from build123d import *

# Parameters (mm, degrees)
F0_R     = 1.905
F1_DEPTH = 38.1
F2_W     = 71.755
F2_H     = 11.43
F2_R     = 1.905
F3_DEPTH = 0.762
F5_DEPTH = 11.43
F6_R     = 0.762


# Not quite as in the source:
# - a feature names something its author has since deleted; it is built from what else it names


with BuildPart() as f1:
    # F0 (on Top) → F1 (new body)
    with BuildSketch(Plane.XY):
        Circle(F0_R)
    extrude(amount=F1_DEPTH)

    # F2 (on face) → F3 (join)
    with BuildSketch(Plane.XY.offset(38.1)):
        Rectangle(F2_W, F2_H)
        Circle(F2_R, mode=Mode.SUBTRACT)
    extrude(amount=-F3_DEPTH)

    # F4 (on face) → F5 (join, through all)
    with BuildSketch(Plane.XZ.offset(5.715)):
        with BuildLine():
            ThreePointArc((0, 46.1144251321), (-18.0910863279, 47.2907715726), (-35.8775, 50.8))
            Line((-35.8775, 50.8), (-35.8775, 48.0069763479))
            ThreePointArc((-35.8775, 48.0069763479), (-23.5669827894, 41.6891623658), (-10.2035430744, 38.1))
            Line((-10.2035430744, 38.1), (0, 38.1))
            Line((0, 38.1), (0, 46.1144251321))
        make_face()
        with BuildLine():
            ThreePointArc((35.8775, 50.8), (18.0910863279, 47.2907715726), (0, 46.1144251321))
            Line((0, 46.1144251321), (0, 38.1))
            Line((0, 38.1), (10.2035430744, 38.1))
            ThreePointArc((10.2035430744, 38.1), (23.5669827894, 41.6891623658), (35.8775, 48.0069763479))
            Line((35.8775, 48.0069763479), (35.8775, 50.8))
        make_face()
    extrude(amount=-F5_DEPTH)

    # F6
    f6_edges = [f1.edges().sort_by_distance(p)[0] for p in [
        (10.203543, 0, 38.1),
        (-10.203543, 0, 38.1),
    ]]
    fillet(f6_edges, radius=F6_R)


solid = f1.part
Work out the finished part from the listing and answer in its coordinate system (mm). A direction names the side the tool comes from. Give positions to 0.01 mm unless a question says otherwise; leave off trailing zeros. Write each loop counter-clockwise with the first axis right and the second up, starting at its lowest first coordinate (ties: lowest second). Pieces come first, ordered by that corner, then holes.
Q1. A tool of negligible diameter and unlimited length cuts with its end or side. For faces 1 (the face through (26.734, -0.08, 43.007)), 2 (the face through (-0.41, -1.86, 18.41)), 3 (the face through (-35.878, 0, 49)), 4 (the face through (-27, 0, 38.1)), from which of +Z, -Z, +X, -X, +Y, -Y can it reach the whole face along a straight path? Write none if from no direction.
Answer:
face 1: +X, +Y, -Y
face 2: -Z
face 3: +Z, -Z, -X, +Y, -Y
face 4: -X, +Y, -Y
Q2. For a pull along Z with two mould halves and no side action, classify faces 5 (the face through (-1, 5.715, 43)), 6 (the face through (16.637, 0.08, 38.746)), 7 (the face through (0, 0, 0)) as released by +Z, released by -Z, zero draft, split by the parting line, or undercut.
Answer:
face 5: zero draft
face 6: undercut
face 7: released by -Z
Q3. The part is cut by section B-B on x = 19. Give the vertices of the cut face in (y, z) (3 decimals).
Answer:
outline: (-5.715, 37.338) - (5.715, 37.338) - (5.715, 38.1) - (-5.715, 38.1) - close; (-5.715, 40.118) - (5.715, 40.118) - (5.715, 47.413) - (-5.715, 47.413) - close
Q4. The part is cut by section D-D on z = 27. Give the vertices of the cut face in (x, y) (3 decimals).
Answer:
outline: circle Ø3.81 at (0, 0)
Q5. The part is cut by section C-C on x = 28. Give the vertices of the cut face in (y, z) (3 decimals).
Answer:
outline: (-5.715, 37.338) - (5.715, 37.338) - (5.715, 38.1) - (-5.715, 38.1) - close; (-5.715, 43.59) - (5.715, 43.59) - (5.715, 48.949) - (-5.715, 48.949) - close
Q6. Given pin 1 (1.5 mm diameter, centred on x = 1.5, z = 22, fed in from -Y); pin 2 (3.5 mm diameter, centred on x = -27, y = -2, fed in from +Z); pin 3 (1.5 mm diameter, centred on x = -23, y = 1.5, fed in from -Z), each flat-ended and moving along its own axis, determine where each tip first touches the part or whether it passes through.
Answer:
pin 1: stops at y = -1.75
pin 2: stops at z = 49.1
pin 3: stops at z = 37.34
Q7. Straight lines are drawn through the part: L1, parallel to Z at x = 2, y = 4; L2, parallel to Z at x = -21.5, y = -2.5; L3, parallel to Z at x = 33, y = 5. For each, find the intervals that lie inside material, in ascending order.
Answer:
L1: z = 37.34 to 46.13
L2: z = 37.34 to 38.1, 40.93 to 47.78
L3: z = 37.34 to 38.1, 46.23 to 50.07
Q8. The part is cut by section A-A on y = 0. Give the vertices of the cut face in (x, z) (1 decimal).
Answer:
outline: (-35.9, 37.3) - (-1.9, 37.3) - (-1.9, 0) - (1.9, 0) - (1.9, 37.3) - (35.9, 37.3) - (35.9, 38.1) - (17.4, 38.1) arc R0.8 cw to (17.2, 39.6) arc R65.5 ccw to (35.9, 48) - (35.9, 50.8) arc R139.7 cw to (-35.9, 50.8) - (-35.9, 48) arc R65.5 ccw to (-17.2, 39.6) arc R0.8 cw to (-17.4, 38.1) - (-35.9, 38.1) - close
